```python
from build123d import *

# Parameters (mm, degrees)
SKETCH1_W           = 105
SKETCH1_H           = 55
SKETCH1_R           = 22.5
SKETCH1_R_2         = 6
SKETCH1_R_3         = 1.5
BOSS_EXTRUDE1_DEPTH = 3


with BuildPart() as part:
    # Sketch1 → Boss-Extrude1 (new body)
    with BuildSketch(Plane(origin=(0, 0, 0), x_dir=(1, 0, 0), z_dir=(0, 1, 0))):
        with Locations((52.5, 27.5)):
            Rectangle(SKETCH1_W, SKETCH1_H)
        with Locations(Location((27.5, 27.5, 0), (0, 0, 270))):
            Circle(SKETCH1_R, mode=Mode.SUBTRACT)
        with Locations(Location((63, 27.5, 0), (0, 0, 270))):
            Circle(SKETCH1_R_2, mode=Mode.SUBTRACT)
        with Locations(Location((4, 4, 0), (0, 0, 270))):
            Circle(SKETCH1_R_3, mode=Mode.SUBTRACT)
        with Locations(Location((51, 4, 0), (0, 0, 270))):
            Circle(SKETCH1_R_3, mode=Mode.SUBTRACT)
        with Locations(Location((51, 51, 0), (0, 0, 270))):
            Circle(SKETCH1_R_3, mode=Mode.SUBTRACT)
        with Locations(Location((4, 51, 0), (0, 0, 270))):
            Circle(SKETCH1_R_3, mode=Mode.SUBTRACT)
        with BuildLine():
            Line((98, 45), (68, 45))
            ThreePointArc((68, 45), (65.5, 47.5), (68, 50))
            Line((68, 50), (98, 50))
            ThreePointArc((98, 50), (100.5, 47.5), (98, 45))
        make_face(mode=Mode.SUBTRACT)
        with BuildLine():
            Line((98, 5), (68, 5))
            ThreePointArc((68, 5), (65.5, 7.5), (68, 10))
            Line((68, 10), (98, 10))
            ThreePointArc((98, 10), (100.5, 7.5), (98, 5))
        make_face(mode=Mode.SUBTRACT)
    extrude(amount=BOSS_EXTRUDE1_DEPTH)


solid = part.part
```
Could you check a few things on this model? Use its own coordinates, in mm. A direction names the side the tool comes from. Round coordinates to 2 decimals unless told otherwise and drop trailing zeros. Write each loop counter-clockwise with the first axis right and the second up, starting at its lowest first coordinate (ties: lowest second). Pieces come first, ordered by that corner, then holes. Notation, with made-up numbers: M 78,31.5 L 122,31.5 A31 ccw 122,59.5 Z; hole C -9,-36 d9. An arc over 180 degrees is marked long. Write each question's results on one line, items separated by ' | '. Start each with the question number.
1. I need wall thicknesses on L1, parallel to Z at x = 90.5, y = 2.85; L2, parallel to X at y = 1.65, z = -51; L3, parallel to X at y = 1.95, z = -27.5. Which ranges of each line are inside material? Lowest first, please. Write a range as from..to.
2. Imagine slicing it at B-B on z = -27.5. List the corners of the cut face in (x, y) for me, and give its area (3 significant figures).
3. On a 3-axis mill with a long thin cutter (end or side, diameter ignored), from which of +Z, -Z, +X, -X, +Y, -Y can I reach the whole of each face in a straight line? I mean faces 4 (the face through (65.5, 1.5, -47.4)), 5 (the face through (63, 3, -34)). Say none if no direction works.
4. Imagine slicing it at D-D on x = 51. List the corners of the cut face in (y, z) for me.
5. Thinking about a two-plate mould opening in Z: for faces 1 (the face through (63.264, 1.479, -33.494)), 2 (the face through (52, 1, -55)), 3 (the face through (63, 0, -34)), which applies, +Z half, -Z half, draft (parallel to the pull), parting line (faces both ways), or undercut?
6. Imagine slicing it at C-C on y = 2. Count the separate pieces of the cut face and the enclosed holes in it, and give its area (3 significant figures).
7. I'm going to push flat-ended pins straight in: pin 1 Ø5 at (x, z) = (4, -51) entering from -Y; pin 2 Ø2.5 at (x, z) = (4, -4) entering from -Y. Where does each tip first touch, or does it pass through?
8. Imagine slicing it at A-A on x = 63. List the corners of the cut face in (y, z) for me, and give its area (3 significant figures).
Result sheet:
1) L1: z = -55..-50, -45..-10, -5..0 | L2: x = 0..2.5, 5.5..49.5, 52.5..105 | L3: x = 0..5, 50..57, 69..105
2) outline: M 0,0 L 5,0 L 5,3 L 0,3 Z; M 50,0 L 57,0 L 57,3 L 50,3 Z; M 69,0 L 105,0 L 105,3 L 69,3 Z | area: 144 mm^2
3) face 4: +Y, -Y | face 5: +Z, -Z, +X, -X, +Y
4) outline: M 0,-55 L 3,-55 L 3,-52.5 L 0,-52.5 Z; M 0,-49.5 L 3,-49.5 L 3,-5.5 L 0,-5.5 Z; M 0,-2.5 L 3,-2.5 L 3,0 L 0,0 Z
5) face 1: undercut | face 2: -Z half | face 3: draft
6) separate pieces: 1 | enclosed holes: 8 | area: 3,700 mm^2
7) pin 1: stops at y = 0 | pin 2: passes through
8) outline: M 0,-55 L 3,-55 L 3,-33.5 L 0,-33.5 Z; M 0,-21.5 L 3,-21.5 L 3,0 L 0,0 Z | area: 129 mm^2
